The model under review builds one solid part; all positions refer to its coordinate system, in mm. Coordinates: 2 decimals unless noted, no trailing zeros. Loops run counter-clockwise (first coordinate to the right, second up) from the corner with the lowest first, then second, coordinate; pieces in that order, holes last. Notation, with made-up numbers: (86, -25) - (115, -25) arc R28 cw to (115, 6) - close; hole circle Ø6 at (33, -1.5). An arc over 180 degrees is marked (long way). One line per item, written item: value. Start each with the question number.
1. We need section B-B, the plane x = -130. Give the boundary of the cut face in (y, z), then the cut area to 3 significant figures.
2. We need section A-A, the plane y = 101.6. Give the boundary of the cut face in (x, z), then the cut area to 3 significant figures.
3. We need section C-C, the plane x = 209. Give the boundary of the cut face in (y, z), then the cut area to 3 significant figures.
4. We need section D-D, the plane z = 510.8. Count the separate pieces of the cut face and the enclosed holes in it, then the cut area to 3 significant figures.
5. To check wall thickness, follow line 1 (Y direction, x = -157, z = 509.2); line 2 (Y direction, x = -162, z = 510.3); line 3 (X direction, y = -111.5, z = 511.1). State the ranges of each line that lie inside material, in increasing order.
from build123d import *

# Parameters (mm, degrees)
F1_R     = 240
F1_R_2   = 12.5
F1_R_3   = 177.8
F2_DEPTH = 3


with BuildPart() as f2:
    # F1 (on offset) → F2 (new body)
    with BuildSketch(Plane.XY.offset(512)):
        with Locations((0, 101.6)):
            Circle(F1_R)
        with Locations((-153.795725, -52.195725)):
            Circle(F1_R_2, mode=Mode.SUBTRACT)
        with Locations((-56.293142, -108.488867)):
            Circle(F1_R_2, mode=Mode.SUBTRACT)
        with Locations((-210.088867, 45.306858)):
            Circle(F1_R_2, mode=Mode.SUBTRACT)
        with Locations((56.293142, -108.488867)):
            Circle(F1_R_2, mode=Mode.SUBTRACT)
        with Locations((153.795725, -52.195725)):
            Circle(F1_R_2, mode=Mode.SUBTRACT)
        with Locations((210.088867, 45.306858)):
            Circle(F1_R_2, mode=Mode.SUBTRACT)
        with Locations((-210.088867, 157.893142)):
            Circle(F1_R_2, mode=Mode.SUBTRACT)
        with Locations((-153.795725, 255.395725)):
            Circle(F1_R_2, mode=Mode.SUBTRACT)
        with Locations((-56.293142, 311.688867)):
            Circle(F1_R_2, mode=Mode.SUBTRACT)
        with Locations((0, 101.6)):
            Circle(F1_R_3, mode=Mode.SUBTRACT)
        with Locations((210.088867, 157.893142)):
            Circle(F1_R_2, mode=Mode.SUBTRACT)
        with Locations((56.293142, 311.688867)):
            Circle(F1_R_2, mode=Mode.SUBTRACT)
        with Locations((153.795725, 255.395725)):
            Circle(F1_R_2, mode=Mode.SUBTRACT)
    extrude(amount=-F2_DEPTH)


solid = f2.part
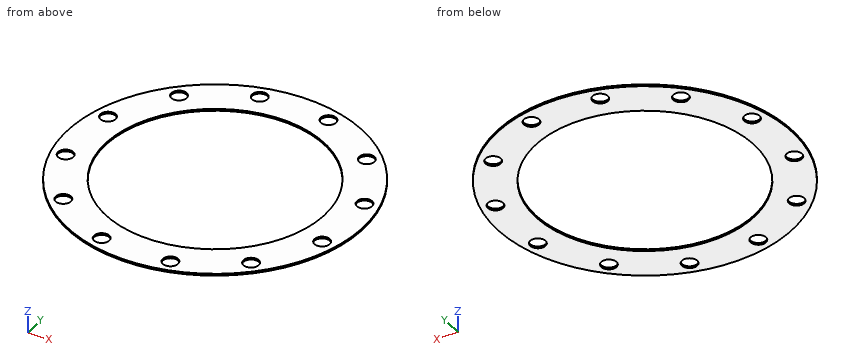
Findings below:
1. outline: (-100.14, 509) - (-19.7, 509) - (-19.7, 512) - (-100.14, 512) - close; (222.9, 509) - (303.34, 509) - (303.34, 512) - (222.9, 512) - close
1. area: 483 mm2
2. outline: (-240, 509) - (-177.8, 509) - (-177.8, 512) - (-240, 512) - close; (177.8, 509) - (240, 509) - (240, 512) - (177.8, 512) - close
2. area: 373 mm2
3. outline: (-16.38, 509) - (32.85, 509) - (32.85, 512) - (-16.38, 512) - close; (57.76, 509) - (145.44, 509) - (145.44, 512) - (57.76, 512) - close; (170.35, 509) - (219.58, 509) - (219.58, 512) - (170.35, 512) - close
3. area: 558 mm2
4. separate pieces: 1
4. enclosed holes: 13
4. area: 75,800 mm2
5. line 1: -79.92 to -64.28, -40.11 to 18.15, 185.05 to 243.31, 267.48 to 283.12
5. line 2: -75.48 to -61.63, -42.76 to 28.33, 174.87 to 245.96, 264.83 to 278.68
5. line 3: -110.4 to -68.43, -44.16 to 44.16, 68.43 to 110.4
